Source: CAD feature listing. Evaluate the final solid. Frame: model axes, mm. Face numbers are marked on the shaded views. A direction names the side the tool comes from. Coordinates: 2 decimals unless noted, no trailing zeros. Loops run counter-clockwise (first coordinate to the right, second up) from the corner with the lowest first, then second, coordinate; pieces in that order, holes last. Notation, with made-up numbers: M -10.75,7.5 L 11.25,7.5 A17 ccw 11.25,12.5 Z; hole C 23,52 d10. An arc over 180 degrees is marked long. One line per question, with ' | ' between items. Start each with the question number.
1. Section query B-B, the plane z = 12. Output: boundary loops of the cut face in (x, y), and give its area (3 significant figures).
2. Section query C-C, the plane z = 7.25. Output: boundary loops of the cut face in (x, y), and give its area (3 significant figures).
3. Section query D-D, the plane x = -11.25. Output: boundary loops of the cut face in (y, z), and give its area (3 significant figures).
4. Mould query, pull axis Z, two halves, no side actions, for the marked faces 1, 2 and 3. Classes: pulls with the +Z half, pulls with the -Z half, needs draft (parallel to the pull), parting line crosses it, or undercut.
5. Section query A-A, the plane x = -19. Output: boundary loops of the cut face in (y, z).
6. Ray query, probe 1 along Z at (x, y) = (-19, 7.9); probe 2 along Z at (x, y) = (-6.5, 2.5); probe 3 along X at (y, z) = (3.5, 11.75). Return the intervals inside material, ascending.
7. Access query for the marked faces 4, 5, 6, 7 and 8. Directions: +Z, -Z, +X, -X, +Y, -Y. A direction counts if a zero-diameter tool reaches every point of the face in a straight line with its end or side. Return the directions, or none.
8. Pin query (flat end, axial travel): P1, Ø2.5, axis at x = 0.5, y = 3.5, coming from the +Z side; P2, Ø1, axis at x = -5.5, z = 9.5, coming from the -Y side; P3, Ø2.5, axis at y = 8.5, z = 8.5, coming from the +X side; P4, Ø2.5, axis at x = -19, z = 11.45, coming from the +Y side. Return the tip coordinate at first contact, or that it passes through.
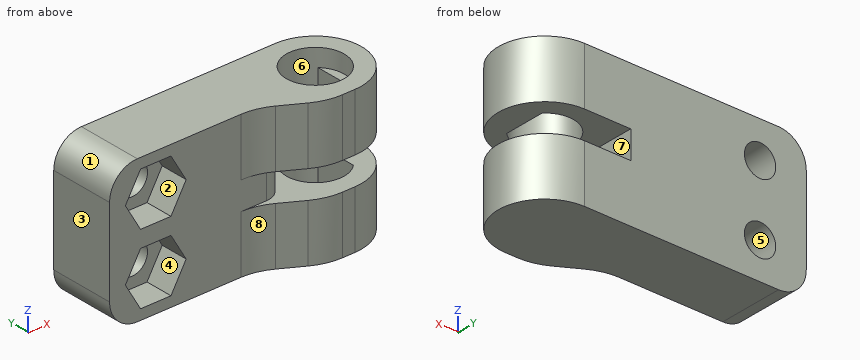
```python
from build123d import *

# Parameters (mm, degrees)
DODANIE_WYCI_GNI_CIE1_DEPTH      = 15.4
SZKIC2_R                         = 3.13
WYTNIJ_WYCI_GNI_CIE1_DEPTH       = 13
WYTNIJ_WYCI_GNI_CIE13_DEPTH      = 7.62
WYTNIJ_WYCI_GNI_CIE13_DEPTH_BACK = 9.78
DODANIE_WYCI_GNI_CIE2_START      = -17.88
DODANIE_WYCI_GNI_CIE2_DEPTH      = 13.5
SZKIC18_W                        = 10
SZKIC18_H                        = 3
WYTNIJ_WYCI_GNI_CIE14_DEPTH      = 11
ZAOKR_GLENIE2_R                  = 3
ZAOKR_GLENIE3_R                  = 6
WYTNIJ_WYCI_GNI_CIE15_DEPTH      = 3
ZAOKR_GLENIE5_R                  = 2
SZKIC20_R                        = 1.7
WYTNIJ_WYCI_GNI_CIE16_DEPTH      = 11
WYTNIJ_WYCI_GNI_CIE17_DEPTH      = 3


with BuildPart() as part:
    # Szkic1 → Dodanie-wyciągnięcie1 (new body)
    with BuildSketch(Plane.XY):
        with BuildLine():
            Line((0, 0), (-24, 0))
            Line((-24, 0), (-24, 10))
            Line((-24, 10), (0, 10))
            ThreePointArc((0, 10), (5, 5), (0, 0))
        make_face()
    extrude(amount=DODANIE_WYCI_GNI_CIE1_DEPTH)

    # Szkic2 → Wytnij-wyciągnięcie1 (cut)
    with BuildSketch(Plane.XY.offset(15.4)):
        with Locations((0, 5)):
            Circle(SZKIC2_R)
    extrude(amount=-WYTNIJ_WYCI_GNI_CIE1_DEPTH, mode=Mode.SUBTRACT)

    # Szkic16 → Wytnij-wyciągnięcie13 (cut, two sides)
    with BuildSketch(Plane(origin=(0, 0, 6.62), x_dir=(-1, 0, 0), z_dir=(0, 0, -1))) as wytnij_wyci_gni_cie13_sk:
        Polygon((31, 0), (31, 3), (8.153065534, 3), (3, 0), align=None)
    extrude(amount=WYTNIJ_WYCI_GNI_CIE13_DEPTH, mode=Mode.SUBTRACT)
    extrude(wytnij_wyci_gni_cie13_sk.sketch, amount=-WYTNIJ_WYCI_GNI_CIE13_DEPTH_BACK, mode=Mode.SUBTRACT)

    # Szkic10 → Dodanie-wyciągnięcie2 (add)
    with BuildSketch(Plane.XY.offset(17.88).offset(DODANIE_WYCI_GNI_CIE2_START)):
        with BuildLine():
            Line((2.2, 7.226409666), (2.2, 2.773590334))
            ThreePointArc((2.2, 2.773590334), (3.13, 5), (2.2, 7.226409666))
        make_face()
    extrude(amount=DODANIE_WYCI_GNI_CIE2_DEPTH)

    # Szkic18 → Wytnij-wyciągnięcie14 (cut, through all)
    with BuildSketch(Plane(origin=(0, 10, 0), x_dir=(1, 0, 0), z_dir=(0, 1, 0))):
        with Locations((0, -7.7)):
            Rectangle(SZKIC18_W, SZKIC18_H)
    extrude(amount=-WYTNIJ_WYCI_GNI_CIE14_DEPTH, mode=Mode.SUBTRACT)

    # Zaokrąglenie2
    zaokr_glenie2_edges = [part.edges().sort_by_distance(p)[0] for p in [
        (-24, 6.5, 0),
        (-24, 6.5, 15.4),
    ]]
    fillet(zaokr_glenie2_edges, radius=ZAOKR_GLENIE2_R)

    # Zaokrąglenie3
    zaokr_glenie3_edges = [part.edges().sort_by_distance(p)[0] for p in [
        (-3, 0, 12.3),
        (-8.153065534, 3, 7.7),
        (-3, 0, 3.1),
    ]]
    fillet(zaokr_glenie3_edges, radius=ZAOKR_GLENIE3_R)

    # Szkic19 → Wytnij-wyciągnięcie15 (cut)
    with BuildSketch(Plane(origin=(0, 0, 9.2), x_dir=(-1, 0, 0), z_dir=(0, 0, -1))):
        Polygon((3.986195456, 3), (13.986195456, 3), (0.751466107, -7.194094716), align=None)
    extrude(amount=WYTNIJ_WYCI_GNI_CIE15_DEPTH, mode=Mode.SUBTRACT)

    # Zaokrąglenie5
    zaokr_glenie5_edges = [part.edges().sort_by_distance(p)[0] for p in [
        (-5, 3, 7.7),
    ]]
    fillet(zaokr_glenie5_edges, radius=ZAOKR_GLENIE5_R)

    # Szkic20 → Wytnij-wyciągnięcie16 (cut, through all)
    with BuildSketch(Plane(origin=(0, 10, 0), x_dir=(1, 0, 0), z_dir=(0, 1, 0))):
        with Locations((-19, -3.95)):
            Circle(SZKIC20_R)
        with Locations((-19, -11.45)):
            Circle(SZKIC20_R)
    extrude(amount=-WYTNIJ_WYCI_GNI_CIE16_DEPTH, mode=Mode.SUBTRACT)

    # Szkic21 → Wytnij-wyciągnięcie17 (cut)
    with BuildSketch(Plane(origin=(0, 3, 0), x_dir=(-1, 0, 0), z_dir=(0, -1, 0))):
        Polygon((15.709103466, -3.95), (17.354551733, -6.8), (20.645448267, -6.8), (22.290896534, -3.95), (20.645448267, -1.1), (17.354551733, -1.1), align=None)
        Polygon((15.709103466, -11.45), (17.354551733, -14.3), (20.645448267, -14.3), (22.290896534, -11.45), (20.645448267, -8.6), (17.354551733, -8.6), align=None)
    extrude(amount=-WYTNIJ_WYCI_GNI_CIE17_DEPTH, mode=Mode.SUBTRACT)


solid = part.part
```
Taken from the geometry:
1) outline: M -24,3 L -21.97,3 L -21.97,6 L -20.61,6 L -20.61,10 L -24,10 Z; M -17.39,6 L -16.03,6 L -16.03,3 L -9.77,3 A6 cw -6.75,2.19 L -4.4,0.81 A6 ccw -1.38,0 L 0,0 A5 ccw 0,10 L -17.39,10 Z; hole M 2.2,2.77 L 2.2,7.23 A3.13 ccw long Z | area: 165 mm^2
2) outline: M -24,3 L -7,3 A2 ccw -5,5 L -5,10 L -24,10 Z | area: 132 mm^2
3) outline: M 3,0 L 10,0 L 10,15.4 L 3,15.4 Z | area: 108 mm^2
4) face 1: pulls with the +Z half | face 2: undercut | face 3: needs draft
5) outline: M 3,0 L 10,0 L 10,2.25 L 6,2.25 L 6,1.1 L 3,1.1 Z; M 3,6.8 L 6,6.8 L 6,5.65 L 10,5.65 L 10,9.75 L 6,9.75 L 6,8.6 L 3,8.6 Z; M 3,14.3 L 6,14.3 L 6,13.15 L 10,13.15 L 10,15.4 L 3,15.4 Z
6) probe 1: 0 to 2.25, 5.65 to 9.75, 13.15 to 15.4 | probe 2: 0 to 6.2, 9.2 to 15.4 | probe 3: -24 to -22.12, -15.88 to -2.75, 2.2 to 4.77
7) face 4: -Y | face 5: +Y, -Y | face 6: +Z | face 7: +X, +Y, -Y | face 8: +Z, -Z, -X, -Y
8) P1: z = 2.4 | P2: y = 1.16 | P3: x = 4.35 | P4: through
